from build123d import *

# Parameters (mm, degrees)
SKETCH1_W           = 190.5
SKETCH1_H           = 76.2
BOSS_EXTRUDE1_DEPTH = 50.8
SKETCH2_W           = 28.67365349
SKETCH2_H           = 76.2
SKETCH2_W_2         = 41.184262463
BOSS_EXTRUDE2_DEPTH = 76.2
FILLET1_R           = 25.4
SKETCH4_W           = 22.86
SKETCH4_H           = 6.35
CUT_EXTRUDE1_DEPTH  = 210.380189247
FILLET2_R           = 2.54
SKETCH5_W           = 63.5
SKETCH5_H           = 60.96
CUT_EXTRUDE3_DEPTH  = 40.64
SKETCH7_W           = 50.8
SKETCH7_H           = 5.08
CUT_EXTRUDE4_DEPTH  = 76.2


with BuildPart() as part:
    # Sketch1 → Boss-Extrude1 (new body)
    with BuildSketch(Plane(origin=(0, 0, 0), x_dir=(1, 0, 0), z_dir=(0, 1, 0))):
        with Locations((8.93730635, -3.65372617)):
            Rectangle(SKETCH1_W, SKETCH1_H)
    extrude(amount=-BOSS_EXTRUDE1_DEPTH)

    # Sketch2 → Boss-Extrude2 (add)
    with BuildSketch(Plane(origin=(0, 0, 0), x_dir=(1, 0, 0), z_dir=(0, 1, 0))):
        with Locations((-71.975866905, -3.65372617)):
            Rectangle(SKETCH2_W, SKETCH2_H)
        with Locations((83.595175119, -3.65372617)):
            Rectangle(SKETCH2_W_2, SKETCH2_H)
    extrude(amount=BOSS_EXTRUDE2_DEPTH)

    # Fillet1
    fillet1_edges = [part.edges().sort_by_distance(p)[0] for p in [
        (104.18730635, -50.8, 3.65372617),
        (-57.63904016, 0, 3.65372617),
        (63.003043887, 0, 3.65372617),
        (-86.31269365, -50.8, 3.65372617),
    ]]
    fillet(fillet1_edges, radius=FILLET1_R)

    # Sketch4 → Cut-Extrude1 (cut, symmetric)
    with BuildSketch(Plane.ZY.offset(86.31269365)):
        with Locations((-17.548825197, 68.000163991)):
            Rectangle(SKETCH4_W, SKETCH4_H)
    cut_extrude1 = extrude(amount=CUT_EXTRUDE1_DEPTH, both=True, mode=Mode.SUBTRACT)

    # Mirror1: Cut-Extrude1 across plane
    add(cut_extrude1.mirror(Plane.XY), mode=Mode.SUBTRACT)

    # Fillet2
    fillet2_edges = [part.edges().sort_by_distance(p)[0] for p in [
        (-86.31269365, 76.2, 3.65372617),
        (-57.63904016, 76.2, 3.65372617),
        (104.18730635, 76.2, 3.65372617),
        (63.003043887, 76.2, 3.65372617),
    ]]
    fillet(fillet2_edges, radius=FILLET2_R)

    # Sketch5 → Cut-Extrude3 (cut)
    with BuildSketch(Plane.XZ.offset(50.8)):
        with Locations((6.612576952, 3.481502269)):
            Rectangle(SKETCH5_W, SKETCH5_H)
    extrude(amount=-CUT_EXTRUDE3_DEPTH, mode=Mode.SUBTRACT)

    # Sketch7 → Cut-Extrude4 (cut)
    with BuildSketch(Plane.ZY.offset(-38.362576952)):
        with Locations((3.329763468, -12.7)):
            Rectangle(SKETCH7_W, SKETCH7_H)
    extrude(amount=-CUT_EXTRUDE4_DEPTH, mode=Mode.SUBTRACT)


solid = part.part
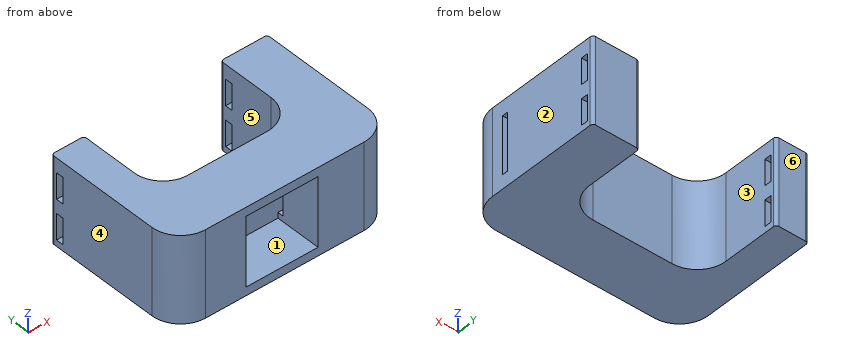
Could you check a few things on this model? Use its own coordinates, in mm. Face numbers are marked on the shaded views. A direction names the side the tool comes from. Give positions to 0.01 mm unless a question says otherwise; leave off trailing zeros. Order: outer loops, then holes, each group sorted by start corner. A loop starts at its lowest first (then second) coordinate and runs counter-clockwise, first axis right, second up.
1. We'd pull the mould along X, two halves only. Please class the marked faces 4, 5 and 6: pulls with the +X half, pulls with the -X half, needs draft (parallel to the pull), parting line crosses it, or undercut.
2. Suppose I cut it at A-A (y = -18.5). List the corners of the cut face in (x, z) for me, plus the area to 3 significant figures.
3. Suppose I cut it at D-D (x = 28.5). List the corners of the cut face in (y, z) for me.
4. I need wall thicknesses on L1, parallel to X at y = 58, z = -4; L2, parallel to X at y = -26, z = -3; L3, parallel to Y at x = 88, z = 21. Which ranges of each line are inside material? Lowest first, please.
5. Will these pins go through, and if not, where does the flat tip stop? P1, Ø2, axis at x = 58.5, z = 27, coming from the +Y side; P2, Ø1, axis at x = -15, z = 32.5, coming from the +Y side; P3, Ø11.5, axis at x = -76.5, z = 15, coming from the -Y side.
6. For the marked faces 1, 2 and 3, which set-ups out of +Z, -Z, +X, -X, +Y, -Y let a thin tool reach every point of the face, with its end or its side?
7. Suppose I cut it at B-B (z = 13). Give the number of separate pieces and of enclosed holes in the cut face, plus the area to 3 significant figures.
8. Suppose I cut it at C-C (y = 39.5). List the corners of the cut face in (x, z) for me, plus the area to 3 significant figures.
Solved:
1. face 4: pulls with the -X half
1. face 5: undercut
1. face 6: needs draft
2. outline: (-86.31, -34.45) - (104.19, -34.45) - (104.19, 41.75) - (-86.31, 41.75) - close; hole (-25.14, -27) - (38.36, -27) - (38.36, 33.96) - (-25.14, 33.96) - close
2. area: 10,600 mm2
3. outline: (-50.8, -34.45) - (0, -34.45) - (0, 41.75) - (-50.8, 41.75) - (-50.8, 33.96) - (-10.16, 33.96) - (-10.16, -27) - (-50.8, -27) - close
4. L1: x = -86.31 to -57.64, 63 to 104.19
4. L2: x = -86.31 to -25.14, 38.36 to 104.18
4. L3: y = -49.07 to -15.24, -10.16 to 64.83, 71.18 to 76.2
5. P1: stops at y = 12.53
5. P2: stops at y = 0
5. P3: stops at y = -48.82
6. face 1: -Y
6. face 2: +Z, -Z, +X, +Y, -Y
6. face 3: +Z, -Z, +Y
7. separate pieces: 4
7. enclosed holes: 0
7. area: 11,600 mm2
8. outline: (-86.31, -34.45) - (-57.64, -34.45) - (-57.64, 41.75) - (-86.31, 41.75) - close; (63, -34.45) - (104.19, -34.45) - (104.19, 41.75) - (63, 41.75) - close
8. area: 5,320 mm2
